```python
from build123d import *

# Parameters (mm, degrees)
F1_DEPTH = 70
F2_W     = 150
F2_H     = 150
F3_DEPTH = 60
F4_W     = 150
F4_H     = 150
F5_DEPTH = 60
F6_R     = 12.5
F7_DEPTH = 400.001


with BuildPart() as f1:
    # F0 (on Front) → F1 (new body)
    with BuildSketch(Plane.XZ):
        Polygon((-200, 0), (-140, 0), (-140, 150), (-100, 190), (100, 190), (140, 150), (140, 0), (200, 0), (200, 174.852814), (124.852814, 250), (-124.852814, 250), (-200, 174.852814), align=None)
    extrude(amount=F1_DEPTH)

    # F2 (on face) → F3 (join, through all)
    with BuildSketch(Plane.YZ.offset(200)):
        with Locations((-35, 0)):
            Rectangle(F2_W, F2_H)
    extrude(amount=-F3_DEPTH)

    # F4 (on face) → F5 (join, through all)
    with BuildSketch(Plane(origin=(-200, 0, 0), x_dir=(0, -1, 0), z_dir=(-1, 0, 0))):
        with Locations((35, 0)):
            Rectangle(F4_W, F4_H)
    extrude(amount=-F5_DEPTH)

    # F6 (on face) → F7 (cut, through all)
    with BuildSketch(Plane.YZ.offset(200)):
        with Locations((-35, 0)):
            Circle(F6_R)
    extrude(amount=-F7_DEPTH, mode=Mode.SUBTRACT)


solid = f1.part
```
The listing builds one solid part. Answer for the finished solid, in the listing's coordinates (mm). A direction names the side the tool comes from. Round coordinates to 2 decimals unless told otherwise and drop trailing zeros. Loops run counter-clockwise (first coordinate to the right, second up) from the corner with the lowest first, then second, coordinate; pieces in that order, holes last.
Q1. Section A-A, the plane z = 45 is taken. Determine the outline of the cut face in (x, y).
Q2. Section C-C, the plane z = 0 is taken. Determine the outline of the cut face in (x, y), then the cut area to 3 significant figures.
Q3. Section B-B, the plane y = -35 is taken. Determine the outline of the cut face in (x, z).
Q4. Find the intervals of material crossed by line 1 (X direction, y = 23, z = -33); line 2 (Z direction, x = -99, y = -22); line 3 (Z direction, x = 161, y = -35), in increasing order.
Q5. For a pull along Z with two mould halves and no side action, classify faces 1 (the face through (-169.58, -44.92, -7.606)), 2 (the face through (120, -35, 170)), 3 (the face through (170, 40, -1)), 4 (the face through (170.42, -44.92, -7.606)) as released by +Z, released by -Z, zero draft, split by the parting line, or undercut.
Q6. Which of the six approach directions +Z, -Z, +X, -X, +Y, -Y give full straight-line access (tool end or side, diameter ignored) to faces 5 (the face through (162.95, -34.51, 211.9)), 6 (the face through (-3, 0, 203)), 7 (the face through (-1, -35, 190)), 8 (the face through (-170, -90, 75))?
Q7. Section D-D, the plane y = 25.5 is taken. Determine the outline of the cut face in (x, z), then the cut area to 3 significant figures.
Q8. Given pin 1 Ø12 at (x, y) = (115.5, -60) entering from -Z; pin 2 Ø20 at (x, y) = (183.5, 17) entering from +Z; pin 3 Ø3 at (x, y) = (-139.5, -31) entering from -Z; pin 4 Ø1 at (x, y) = (39, -14.5) entering from -Z, each flat-ended and moving along its own axis, determine where each tip first touches the part or whether it passes through.
Completed:
1. outline: (-200, -110) - (-140, -110) - (-140, 40) - (-200, 40) - close; (140, -110) - (200, -110) - (200, 40) - (140, 40) - close
2. outline: (-200, -110) - (-140, -110) - (-140, -47.5) - (-200, -47.5) - close; (-200, -22.5) - (-140, -22.5) - (-140, 40) - (-200, 40) - close; (140, -110) - (200, -110) - (200, -47.5) - (140, -47.5) - close; (140, -22.5) - (200, -22.5) - (200, 40) - (140, 40) - close
2. area: 15,000 mm2
3. outline: (-200, -75) - (-140, -75) - (-140, -12.5) - (-200, -12.5) - close; (-200, 12.5) - (-140, 12.5) - (-140, 150) - (-100, 190) - (100, 190) - (140, 150) - (140, 12.5) - (200, 12.5) - (200, 174.85) - (124.85, 250) - (-124.85, 250) - (-200, 174.85) - close; (140, -75) - (200, -75) - (200, -12.5) - (140, -12.5) - close
4. line 1: x = -200 to -140, 140 to 200
4. line 2: z = 190 to 250
4. line 3: z = -75 to -12.5, 12.5 to 213.85
5. face 1: undercut
5. face 2: released by -Z
5. face 3: zero draft
5. face 4: undercut
6. face 5: +Z, +X, +Y, -Y
6. face 6: +Z, +X, -X, +Y
6. face 7: -Z, +Y, -Y
6. face 8: +Z, +X, -X, -Y
7. outline: (-200, -75) - (-140, -75) - (-140, 75) - (-200, 75) - close; (140, -75) - (200, -75) - (200, 75) - (140, 75) - close
7. area: 18,000 mm2
8. pin 1: stops at z = 168.5
8. pin 2: stops at z = 75
8. pin 3: stops at z = -75
8. pin 4: stops at z = 190
